```python
from build123d import *

# Parameters (mm, degrees)
F1_DEPTH = 80
F2_W     = 30
F2_H     = 25
F3_DEPTH = 80.001
F4_R     = 2


# Not quite as in the source:
# - a feature names something its author has since deleted; it is built from what else it names


with BuildPart() as f1:
    # F0 (on Front) → F1 (new body)
    with BuildSketch(Plane.XZ):
        with BuildLine():
            Line((112.9777067155, -18.5589175671), (112.9777067155, 31.4410824329))
            ThreePointArc((112.9777067155, 31.4410824329), (99.260783713, 40.7246422778), (95.7408100367, 24.5398270065))
            Line((95.7408100367, 24.5398270065), (95.7408100367, 21.3474755859))
            Line((95.7408100367, 21.3474755859), (50.9332562928, 21.3474755859))
            Line((50.9332562928, 21.3474755859), (50.9332562928, 14.1588503625))
            Line((50.9332562928, 14.1588503625), (-7.0222932845, -8.5589175671))
            Line((-7.0222932845, -8.5589175671), (-7.0222932845, -18.5589175671))
            Line((-7.0222932845, -18.5589175671), (112.9777067155, -18.5589175671))
        make_face()
    extrude(amount=F1_DEPTH)

    # F2 (on face) → F3 (cut, through all)
    with BuildSketch(Plane.XZ.offset(80)):
        with Locations((77.9777067155, -6.0589175671)):
            Rectangle(F2_W, F2_H)
    extrude(amount=-F3_DEPTH, mode=Mode.SUBTRACT)

    # F4
    f4_edges = [f1.edges().sort_by_distance(p)[0] for p in [
        (73.337033, -80, 21.347476),
        (95.74081, -80, 22.943651),
        (99.260784, -80, 40.724642),
        (92.977707, -80, -6.058918),
        (77.977707, -80, 6.441082),
        (62.977707, -80, -6.058918),
        (50.933256, -80, 17.753163),
        (50.933256, -40, 21.347476),
        (73.337033, 0, 21.347476),
        (-7.022293, 0, -13.558918),
        (62.977707, 0, -6.058918),
        (77.977707, 0, 6.441082),
        (92.977707, 0, -6.058918),
        (95.74081, 0, 22.943651),
        (99.260784, 0, 40.724642),
        (-7.022293, -80, -13.558918),
        (-7.022293, -40, -8.558918),
        (-7.022293, -40, -18.558918),
        (50.933256, -40, 14.15885),
        (21.955482, -80, 2.799966),
        (112.977707, 0, 6.441082),
        (112.977707, -80, 6.441082),
    ]]
    fillet(f4_edges, radius=F4_R)


solid = f1.part
```
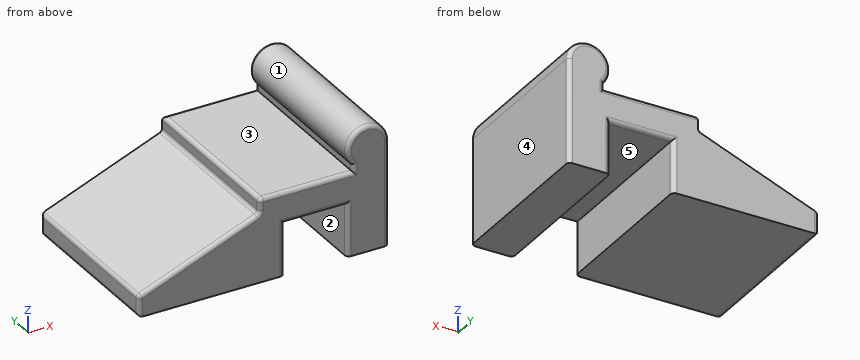
Source: CAD feature listing. Evaluate the final solid. Frame: model axes, mm. Face numbers are marked on the shaded views. A direction names the side the tool comes from. Give positions to 0.01 mm unless a question says otherwise; leave off trailing zeros. Write each loop counter-clockwise with the first axis right and the second up, starting at its lowest first coordinate (ties: lowest second). Pieces come first, ordered by that corner, then holes.
1. Section query B-B (y = -16). Return the cut outline in (x, z), then the cut area to 3 significant figures.
2. Section query A-A (z = -11.5). Return the cut outline in (x, y), then the cut area to 3 significant figures.
3. Material intervals for line 1 along X through (y, z) = (-57, -14); line 2 along Z through (x, y) = (54, -33); line 3 along X through (y, z) = (-21.5, 23.5), sorted ascending.
4. Access query for the marked faces 4 and 5. Directions: +Z, -Z, +X, -X, +Y, -Y. A direction counts if a zero-diameter tool reaches every point of the face in a straight line with its end or side. Return the directions, or none.
5. Section query C-C (x = 76). Return the cut outline in (y, z).
6. Pull-direction query (X, two-part tool) for the marked faces 1, 2 and 3; classes: +X half, -X half, draft (parallel to the pull), parting line (faces both ways), or undercut.
7. First-contact query: pin 1 (3.5 mm diameter, centred on y = -23, z = 22.5, fed in from -X); pin 2 (3 mm diameter, centred on y = -49, z = 18.5, fed in from -X); pin 3 (1.5 mm diameter, centred on y = -10.5, z = 32.5, fed in from -X). Flat tips, straight axial feed; report the tip coordinate or a pass-through.
Output values:
1. outline: (-7.02, -16.56) arc R2 ccw to (-5.02, -18.56) - (62.98, -18.56) - (62.98, 6.44) - (92.98, 6.44) - (92.98, -18.56) - (112.98, -18.56) - (112.98, 31.44) arc R10 ccw (long way) to (95.74, 24.54) - (95.74, 21.35) - (52.93, 21.35) arc R2 ccw to (50.93, 19.35) - (50.93, 15.52) arc R2 cw to (49.66, 13.66) - (-5.75, -8.06) arc R2 ccw to (-7.02, -9.92) - close
1. area: 3,310 mm2
2. outline: (-7.02, -78) arc R2 ccw to (-5.02, -80) - (60.98, -80) arc R2 ccw to (62.98, -78) - (62.98, -2) arc R2 ccw to (60.98, 0) - (-5.02, 0) arc R2 ccw to (-7.02, -2) - close; (92.98, -78) arc R2 ccw to (94.98, -80) - (110.98, -80) arc R2 ccw to (112.98, -78) - (112.98, -2) arc R2 ccw to (110.98, 0) - (94.98, 0) arc R2 ccw to (92.98, -2) - close
2. area: 7,190 mm2
3. line 1: x = -7.02 to 62.98, 92.98 to 112.98
3. line 2: z = -18.56 to 21.35
3. line 3: x = 95.74 to 112.98
4. face 4: +Z, -Z, +X, +Y, -Y
4. face 5: -Z, +Y, -Y
5. outline: (-80, 8.44) arc R2 ccw to (-78, 6.44) - (-2, 6.44) arc R2 ccw to (0, 8.44) - (0, 19.35) arc R2 ccw to (-2, 21.35) - (-78, 21.35) arc R2 ccw to (-80, 19.35) - close
6. face 1: parting line
6. face 2: undercut
6. face 3: draft
7. pin 1: stops at x = 51.51
7. pin 2: stops at x = 50.93
7. pin 3: stops at x = 92.98
